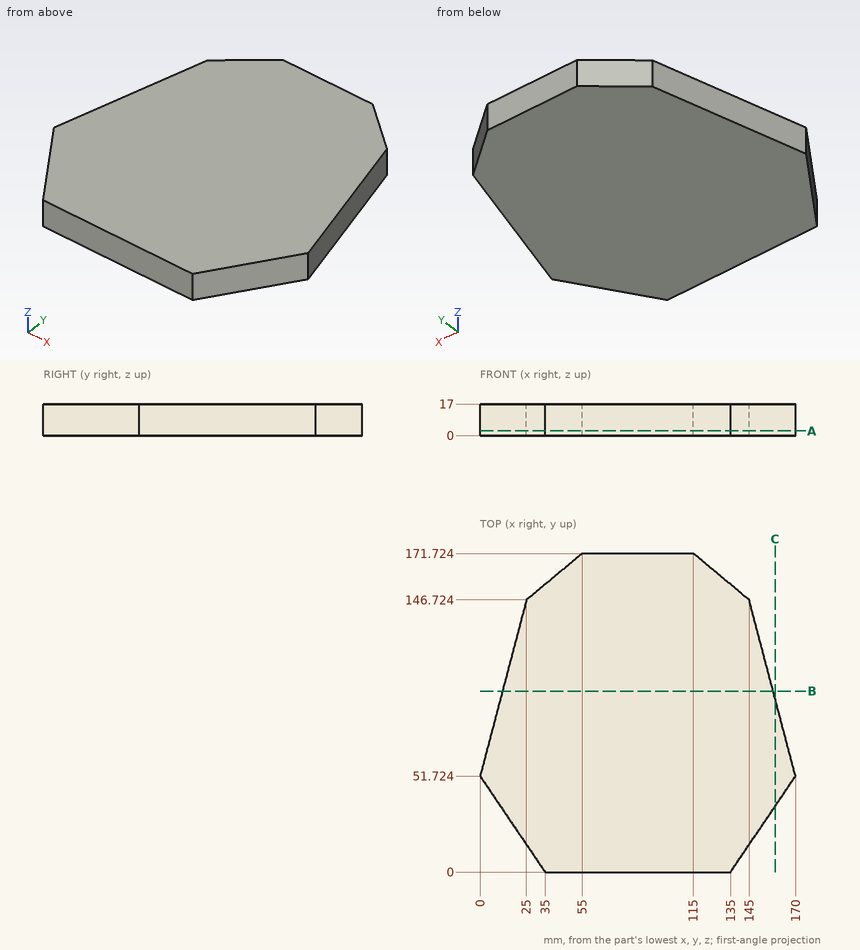
Input: dimensioned drawing with shaded views. Units: mm. Origin: part minimum x, y, z. Round coordinates to 2 decimals unless told otherwise and drop trailing zeros. Loops run counter-clockwise (first coordinate to the right, second up) from the corner with the lowest first, then second, coordinate; pieces in that order, holes last.
1) Material intervals for line 1 (X direction, y = 89.5, z = 12); line 2 (X direction, y = 16.5, z = 1) (1 decimal); line 3 (Y direction, x = 119.5, z = 14.75) (1 decimal), sorted ascending.
Ans:
line 1: x = 9.94 to 160.06
line 2: x = 23.8 to 146.2
line 3: y = 0 to 168
2) Section query A-A on z = 2.5. Return the cut outline in (x, y).
Ans:
outline: (0, 51.72) - (35, 0) - (135, 0) - (170, 51.72) - (145, 146.72) - (115, 171.72) - (55, 171.72) - (25, 146.72) - close
3) Section query B-B on y = 97.5. Return the cut outline in (x, z).
Ans:
outline: (12.05, 0) - (157.95, 0) - (157.95, 17) - (12.05, 17) - close
4) Pin query (flat end, axial travel): pin 1 (8 mm diameter, centred on x = 123, z = 4, fed in from +Y); pin 2 (8 mm diameter, centred on y = 94.5, z = 14.5, fed in from +X); pin 3 (10 mm diameter, centred on y = 139, z = 5, fed in from -X). Return the tip coordinate at first contact, or that it passes through.
Ans:
pin 1: stops at y = 168.39
pin 2: stops at x = 159.8
pin 3: stops at x = 21.65
5) Section query C-C on x = 159. Return the cut outline in (y, z), plus the area to 3 significant figures.
Ans:
outline: (35.47, 0) - (93.52, 0) - (93.52, 17) - (35.47, 17) - close
area: 987 mm2
